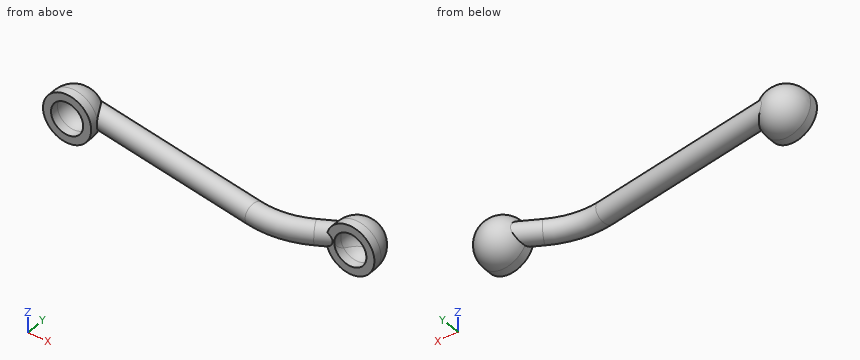
```python
from build123d import *
from build123d.topology import SkipClean

# Parameters (mm, degrees)
SKETCH1_R             = 2.85
SKETCH1_R_2           = 1.9
BOSS_EXTRUDE1_DEPTH   = 1
BOSS_EXTRUDE1_2_DEPTH = 1
SKETCH6_R             = 1.25


with BuildPart() as part:
    # Sketch1 → Boss-Extrude1 (new body)
    with BuildSketch(Plane(origin=(0, 0, 0), x_dir=(1, 0, 0), z_dir=(0, 1, 0))):
        with Locations(Location((2.85, 0, 0), (0, 0, 270))):
            Circle(SKETCH1_R)
        with Locations(Location((2.85, 0, 0), (0, 0, 270))):
            Circle(SKETCH1_R_2, mode=Mode.SUBTRACT)
    extrude(amount=BOSS_EXTRUDE1_DEPTH)

    # Sketch2 → Revolve1 (revolve)
    with BuildSketch(Plane.XY):
        with BuildLine():
            Line((0.95, 1), (0, 1))
            ThreePointArc((0, 1), (0.834745674, 3.015254326), (2.85, 3.85))
            Line((2.85, 3.85), (2.85, 2.9))
            ThreePointArc((2.85, 2.9), (1.506497116, 2.343502884), (0.95, 1))
        make_face()
    revolve(axis=Axis((2.85, 3.85, 0), (0, -1, 0)))



with BuildPart() as body_2:
    # Sketch1 → Boss-Extrude1 2 (new body)
    with BuildSketch(Plane(origin=(0, 0, 0), x_dir=(1, 0, 0), z_dir=(0, 1, 0))):
        with Locations(Location((36.35, 0, 0), (0, 0, 270))):
            Circle(SKETCH1_R)
        with Locations(Location((36.35, 0, 0), (0, 0, 270))):
            Circle(SKETCH1_R_2, mode=Mode.SUBTRACT)
    extrude(amount=BOSS_EXTRUDE1_2_DEPTH)

    # Sketch3 → Revolve2 (revolve)
    with BuildSketch(Plane.XY):
        with BuildLine():
            Line((34.45, 1), (33.5, 1))
            ThreePointArc((33.5, 1), (34.334745674, 3.015254326), (36.35, 3.85))
            Line((36.35, 3.85), (36.35, 2.9))
            ThreePointArc((36.35, 2.9), (35.006497116, 2.343502884), (34.45, 1))
        make_face()
    revolve(axis=Axis((36.35, 3.85, 0), (0, -1, 0)))


with BuildPart() as part_1:
    add(part.part)

    add(body_2.part)  # Sweep2 merges body 2
    # Sweep2: sweep along a path in Sketch4
    with BuildLine(Plane.XY) as sweep2_path:
        Line((2.857791508, 2.577073997), (25.735308166, -0.910058828))
        ThreePointArc((25.735308166, -0.910058828), (29.000921957, -0.868365637), (32.078947298, 0.223299034))
        Line((32.078947298, 0.223299034), (36.338250501, 2.577073997))
    # Sketch6 → Sweep2 (sweep)
    with BuildSketch(Plane(origin=(2.857791508, 2.577073997, 0), x_dir=(0, 0, -1), z_dir=(0.9885817138183747, -0.1506857495051383, 0))):
        Circle(SKETCH6_R)
    sweep(path=sweep2_path.line)

    # Sketch2<3> → Cut-Revolve2 (revolve, cut)
    with BuildSketch(Plane.XY, mode=Mode.PRIVATE) as cut_revolve2_sk:
        with BuildLine():
            ThreePointArc((0.95, 1), (1.506497116, 2.343502884), (2.85, 2.9))
            Line((2.85, 2.9), (2.85, 0))
            Line((2.85, 0), (0.95, 0))
            Line((0.95, 0), (0.95, 1))
        make_face()
    revolve(cut_revolve2_sk.sketch.rotate(Axis((2.85, 2.9, 0), (0, -1, 0)), 169.541612369), axis=Axis((2.85, 2.9, 0), (0, -1, 0)), mode=Mode.SUBTRACT)

    # Sketch3<3> → Cut-Revolve3 (revolve, cut)
    with SkipClean():  # the faces are left unmerged after this step: merging them gives an invalid solid
        with BuildSketch(Plane.XY):
            with BuildLine():
                ThreePointArc((34.45, 1), (35.006497116, 2.343502884), (36.35, 2.9))
                Line((36.35, 2.9), (36.35, 0))
                Line((36.35, 0), (34.45, 0))
                Line((34.45, 0), (34.45, 1))
            make_face()
        revolve(axis=Axis((36.35, 2.9, 0), (0, -1, 0)), mode=Mode.SUBTRACT)


solid = part_1.part
```
Build history of the part. All positions in model axes, mm. Round coordinates to 2 decimals unless told otherwise and drop trailing zeros. Write each loop counter-clockwise with the first axis right and the second up, starting at its lowest first coordinate (ties: lowest second). Pieces come first, ordered by that corner, then holes.
1) Band-saw the part on A-A, the plane z = 0. List the corners of the cut face in (x, y), and give its area (3 significant figures).
2) Drill centre lines: probe 1 along Z at (x, y) = (36.35, 0.45); probe 2 along X at (y, z) = (2.25, -1.65); probe 3 along Z at (x, y) = (35, 1.75). Where is each one in solid material? Low to high.
3) Pin check, flat tips, straight feed: pin 1 (1.5 mm diameter, centred on x = 11.5, y = 2, fed in from +Z); pin 2 (1.5 mm diameter, centred on x = 22.5, y = 1, fed in from -Z); pin 3 (3 mm diameter, centred on x = 14.5, y = 2.5, fed in from -Z). Stop position of each tip, or through.
Ans:
1. outline: (0, 0) - (0.95, 0) - (0.95, 1) arc R1.9 cw to (4.75, 1) - (4.75, 0) - (5.7, 0) - (5.7, 0.88) - (25.55, -2.15) arc R11.25 ccw to (32.68, -0.87) - (34.26, 0) - (34.45, 0) - (34.45, 1) arc R1.9 cw to (38.25, 1) - (38.25, 0) - (39.2, 0) - (39.2, 1) arc R2.85 ccw to (34.13, 2.78) - (31.47, 1.32) arc R8.75 cw to (25.92, 0.33) - (3.74, 3.71) arc R2.85 ccw to (0, 1) - close
1. area: 90.6 mm2
2. probe 1: z = -2.85 to -1.9, 1.9 to 2.85
2. probe 2: x = 0.89 to 4.81, 34.39 to 38.31
2. probe 3: z = -2.4 to -1.11, 1.11 to 2.4
3. pin 1: stops at z = 1.25
3. pin 2: stops at z = -1.07
3. pin 3: stops at z = -1.24
